```python
from build123d import *

# Parameters (mm, degrees)
ESQUISSE1_R               = 1.5
ESQUISSE1_R_2             = 1.25
T_LE_DE_BASE_PLI_E1_DEPTH = 3


# Sheet-metal steps are written as plain solids
with BuildPart() as part:
    # Esquisse1 → Tôle de base pliée1 (new body)
    with BuildSketch(Plane.XY):
        with BuildLine():
            Line((1180.806329324, 1712.423223535), (1163.94410285, 1713.60971993))
            ThreePointArc((1163.94410285, 1713.60971993), (1162.76612345, 1713.612955968), (1161.59842695, 1713.457614973))
            ThreePointArc((1161.59842695, 1713.457614973), (1158.418396897, 1709.091687704), (1162.488835778, 1705.54127373))
            ThreePointArc((1162.488835778, 1705.54127373), (1165.059310496, 1704.535149371), (1166.141947966, 1701.995952134))
            ThreePointArc((1166.141947966, 1701.995952134), (1167.040054527, 1699.743489734), (1169.229884323, 1698.701939096))
            Line((1169.229884323, 1698.701939096), (1179.646505762, 1697.968982283))
            ThreePointArc((1179.646505762, 1697.968982283), (1180.450889379, 1698.077491546), (1181.145910596, 1698.496720327))
            ThreePointArc((1181.145910596, 1698.496720327), (1184.248383676, 1704.858228491), (1182.250729268, 1711.648184471))
            ThreePointArc((1182.250729268, 1711.648184471), (1181.611578951, 1712.190479321), (1180.806329324, 1712.423223535))
        make_face()
        with Locations((1162.31301042, 1709.771535786)):
            Circle(ESQUISSE1_R, mode=Mode.SUBTRACT)
        with Locations((1180.453067935, 1708.517601578)):
            Circle(ESQUISSE1_R_2, mode=Mode.SUBTRACT)
    extrude(amount=-T_LE_DE_BASE_PLI_E1_DEPTH)


solid = part.part
```
Geometry check sheet. Reference: the model listing, model coordinates, mm. Coordinates: 2 decimals unless noted, no trailing zeros. Order: outer loops, then holes, each group sorted by start corner. A loop starts at its lowest first (then second) coordinate and runs counter-clockwise, first axis right, second up. Notation, with made-up numbers: M 20.25,86 L 68.25,86 A24 cw 68.25,121 Z; hole C -25.5,-27.5 d9. An arc over 180 degrees is marked long. Answer as a JSON object with one key per item and string values.
Q1. Cross-section at A-A on z = -2.3. Record the cut outline in (x, y).
Results are:
{"outline": "M 1161.6,1713.46 A4 ccw 1162.49,1705.54 A3.57 cw 1166.14,1702 A3.32 ccw 1169.23,1698.7 L 1179.65,1697.97 A2 ccw 1181.15,1698.5 A9.79 ccw 1182.25,1711.65 A2 ccw 1180.81,1712.42 L 1163.94,1713.61 A8.73 ccw Z; hole C 1162.31,1709.77 d3; hole C 1180.45,1708.52 d2.5"}
Q2. Depth check by flat-ended pin: pin 1 Ø1.5 at (x, y) = (1180.45, 1708.52) entering from -Z. Enter the tip coordinate at first touch or a pass-through.
Results are:
{"pin 1": "passes through"}
Q3. Scan lines: line 1 (X direction, y = 1708.75, z = -0.5); line 2 (Y direction, x = 1175.25, z = -2.35); line 3 (Y direction, x = 1162.25, z = -1.65). Record each from-to range of solid material in increasing order.
Results are:
{"line 1": "x = 1158.47 to 1161.21, 1163.41 to 1179.22, 1181.68 to 1183.79", "line 2": "y = 1698.28 to 1712.81", "line 3": "y = 1705.54 to 1708.27, 1711.27 to 1713.56"}
Q4. Cross-section at B-B on y = 1701.5. Record the cut outline in (x, z), and give its area (3 significant figures).
Results are:
{"outline": "M 1166.18,-3 L 1183.35,-3 L 1183.35,0 L 1166.18,0 Z", "area": "51.5 mm²"}
Q5. Release check for a two-part mould opening along Y. For faces 1 (the flat face through (1171, 1706, -3)), 2 (the cylindrical face through (1180.29, 1709.757, -1.479)), 3 (the cylindrical face through (1181.622, 1712.185, -1.479)) record: released by +Y, released by -Y, zero draft, split by the parting line, or undercut.
Results are:
{"face 1": "zero draft", "face 2": "undercut", "face 3": "released by +Y"}
Q6. Cross-section at C-C on x = 1175.5. Record the cut outline in (y, z).
Results are:
{"outline": "M 1698.26,-3 L 1712.8,-3 L 1712.8,0 L 1698.26,0 Z"}
